The drawing under review shows one solid part. Ordinate dimensions are in mm from its lowest x, y, z. A direction names the side the tool comes from. Coordinates: 2 decimals unless noted, no trailing zeros. Order: outer loops, then holes, each group sorted by start corner. A loop starts at its lowest first (then second) coordinate and runs counter-clockwise, first axis right, second up. Notation, with made-up numbers: M 37,-14.5 L 85,-14.5 A14 ccw 85,8.5 Z; hole C 28,71.5 d1. An arc over 180 degrees is marked long. Answer as a JSON object with one key per item and string values.
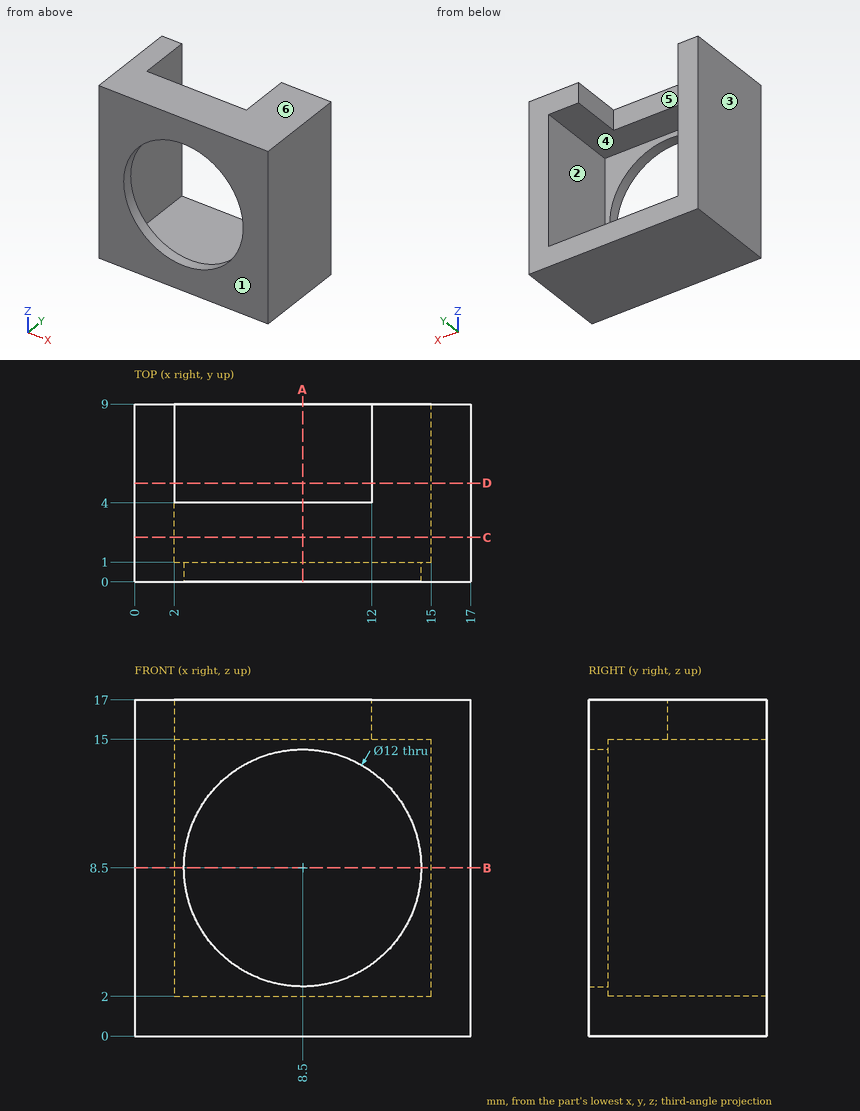
1) Insertion check: pin 1 Ø1.5 at (x, z) = (14, 14) entering from +Y; pin 2 Ø1 at (x, z) = (8.5, 16) entering from +Y; pin 3 Ø2 at (x, z) = (9, 2) entering from -Y. Each pin has a flat end and moves straight along its axis. Give the tip position at first contact, or say it passes through.
Taken from the geometry:
{"pin 1": "stops at y = 1", "pin 2": "stops at y = 4", "pin 3": "stops at y = 0"}
2) Add section C-C (y = 2.25). State the section outline as (x, z) points.
Taken from the geometry:
{"outline": "M 0,0 L 17,0 L 17,17 L 0,17 Z; hole M 2,2 L 15,2 L 15,15 L 2,15 Z"}
3) Tool access review of the marked faces 1 and 2: name each direction out of +Z, -Z, +X, -X, +Y, -Y from which nothing blocks a thin tool from reaching the whole face with its end or side.
Taken from the geometry:
{"face 1": "+Z, -Z, +X, -X, -Y", "face 2": "+Y"}
4) To check wall thickness, follow L1, parallel to Z at x = 2.5, y = 2.5; L2, parallel to Z at x = 8.5, y = 0.45. State the ranges of each line that lie inside material, in increasing order.
Taken from the geometry:
{"L1": "z = 0 to 2, 15 to 17", "L2": "z = 0 to 2.5, 14.5 to 17"}
5) Mouldability with a two-part tool opening along X and no side actions: class the marked faces 3, 4, 5 and 6 as released by +X, released by -X, zero draft, split by the parting line, or undercut.
Taken from the geometry:
{"face 3": "released by -X", "face 4": "undercut", "face 5": "undercut", "face 6": "zero draft"}
6) Add section B-B (z = 8.5). State the section outline as (x, y) points.
Taken from the geometry:
{"outline": "M 0,0 L 2.5,0 L 2.5,1 L 2,1 L 2,9 L 0,9 Z; M 14.5,0 L 17,0 L 17,9 L 15,9 L 15,1 L 14.5,1 Z"}
7) Add section D-D (y = 5). State the section outline as (x, z) points.
Taken from the geometry:
{"outline": "M 0,0 L 17,0 L 17,17 L 12,17 L 12,15 L 15,15 L 15,2 L 2,2 L 2,17 L 0,17 Z"}
8) Add section A-A (x = 8.5). State the section outline as (y, z) points.
Taken from the geometry:
{"outline": "M 0,0 L 9,0 L 9,2 L 1,2 L 1,2.5 L 0,2.5 Z; M 0,14.5 L 1,14.5 L 1,15 L 4,15 L 4,17 L 0,17 Z"}
